Read the model definition and answer for the solid it produces. Units are mm, in the model's axes. Coordinates: 2 decimals unless noted, no trailing zeros. Write each loop counter-clockwise with the first axis right and the second up, starting at its lowest first coordinate (ties: lowest second). Pieces come first, ordered by that corner, then holes.
(1) Straight lines are drawn through the part: line 1 along Y through (x, z) = (-27.5, -25); line 2 along X through (y, z) = (-46, 16); line 3 along X through (y, z) = (-7.5, 15.5). For each, find the intervals that lie inside material, in ascending order.
(2) The part is cut by section C-C, the plane y = -118.5. Determine the outline of the cut face in (x, z), and give its area (3 significant figures).
(3) The part is cut by section A-A, the plane z = -6.5. Determine the outline of the cut face in (x, y).
(4) The part is cut by section B-B, the plane x = -47. Determine the outline of the cut face in (y, z).
(5) Given pin 1 (1 mm diameter, centred on x = -30.5, z = -22, fed in from -Y); pin 2 (6 mm diameter, centred on y = -15.5, z = -13, fed in from -X); pin 3 (5 mm diameter, centred on x = -14, z = -27.5, fed in from +Y), each flat-ended and moving along its own axis, determine where each tip first touches the part or whether it passes through.
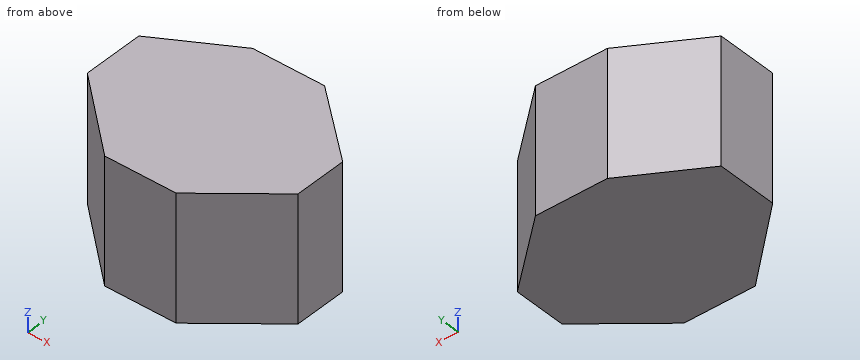
```python
from build123d import *

# Parameters (mm, degrees)
F0_W     = 164.485968
F0_H     = 93.735796
F1_DEPTH = 131.064
F3_DEPTH = 109.474
F5_DEPTH = 175.768
F7_DEPTH = 175.514
F9_DEPTH = 113.538


with BuildPart() as f1:
    # F0 (on Front) → F1 (new body)
    with BuildSketch(Plane.XZ):
        with Locations((16.512107, -18.227907)):
            Rectangle(F0_W, F0_H)
    extrude(amount=F1_DEPTH)

    # F2 (on face) → F3 (cut)
    with BuildSketch(Plane.XY.offset(28.639991)):
        Polygon((-8.129642, -131.064), (-65.730877, -78.621335), (-65.730877, -131.064), align=None)
    extrude(amount=-F3_DEPTH, mode=Mode.SUBTRACT)

    # F4 (on face) → F5 (cut)
    with BuildSketch(Plane.XY.offset(28.639991)):
        Polygon((-65.730877, 0), (-65.730877, -33.21651), (-19.07178, 0), align=None)
    extrude(amount=-F5_DEPTH, mode=Mode.SUBTRACT)

    # F6 (on face) → F7 (cut)
    with BuildSketch(Plane.XY.offset(28.639991)):
        Polygon((-65.730877, -33.21651), (-8.77298, 0), (-19.07178, 0), align=None)
    extrude(amount=-F7_DEPTH, mode=Mode.SUBTRACT)

    # F8 (on face) → F9 (cut)
    with BuildSketch(Plane.XY.offset(28.639991)):
        Polygon((98.755091, 0), (44.991056, 0), (98.755091, -47.293574), align=None)
        Polygon((98.755091, -131.064), (98.755091, -86.671993), (45.312725, -131.064), align=None)
    extrude(amount=-F9_DEPTH, mode=Mode.SUBTRACT)


solid = f1.part
```
Computed:
1. line 1: y = -113.43 to -10.92
1. line 2: x = -65.73 to 97.28
1. line 3: x = -21.63 to 53.52
2. outline: (-21.93, -65.1) - (60.44, -65.1) - (60.44, 28.64) - (-21.93, 28.64) - close
2. area: 7,720 mm2
3. outline: (-65.73, -78.62) - (-8.13, -131.06) - (45.31, -131.06) - (98.76, -86.67) - (98.76, -47.29) - (44.99, 0) - (-8.77, 0) - (-65.73, -33.22) - close
4. outline: (-95.67, -65.1) - (-22.29, -65.1) - (-22.29, 28.64) - (-95.67, 28.64) - close
5. pin 1: stops at y = -111.15
5. pin 2: stops at x = -40.5
5. pin 3: stops at y = -1.59
